For this review, take the finished solid that the model builds, in its own axes (mm). Face numbers are marked on the shaded views. A direction names the side the tool comes from. Give positions to 0.01 mm unless a question says otherwise; leave off trailing zeros. Order: outer loops, then holes, each group sorted by start corner. A loop starts at its lowest first (then second) coordinate and runs counter-clockwise, first axis right, second up.
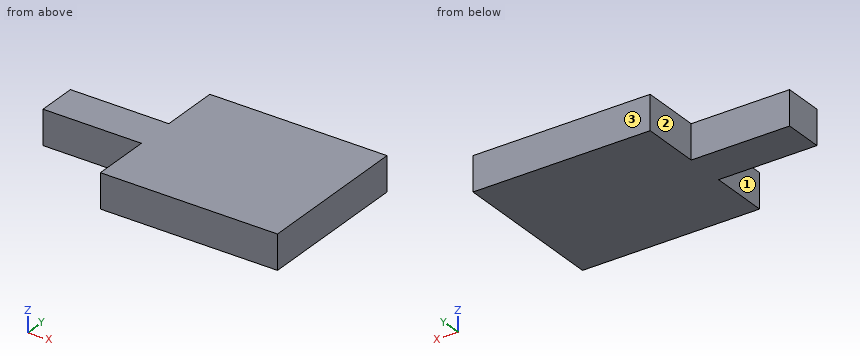
from build123d import *

# Parameters (mm, degrees)
F0_W          = 127
F0_H          = 50.8
F1_DEPTH      = 25.4
F1_DEPTH_BACK = 19.05


with BuildPart() as f1:
    # F0 (on Top) → F1 (new body, two sides)
    with BuildSketch(Plane.XY) as f1_sk:
        Polygon((0, 76.2), (0, 0), (228.6, 0), (228.6, 203.2), (0, 203.2), (0, 127), align=None)
        with Locations((-63.5, 101.6)):
            Rectangle(F0_W, F0_H)
    extrude(amount=F1_DEPTH)
    extrude(f1_sk.sketch, amount=-F1_DEPTH_BACK)


solid = f1.part
1) We need section C-C on y = 65.5. Give the boundary of the cut face in (x, z), then the cut area to 3 significant figures.
Answer sheet:
outline: (0, -19.05) - (228.6, -19.05) - (228.6, 25.4) - (0, 25.4) - close
area: 10,200 mm2
2) To check wall thickness, follow line 1 (X direction, y = 30.5, z = 12); line 2 (Y direction, x = -106.5, z = -5). State the ranges of each line that lie inside material, in increasing order.
Answer sheet:
line 1: x = 0 to 228.6
line 2: y = 76.2 to 127
3) We need section B-B on x = -20.5. Give the boundary of the cut face in (y, z), then the cut area to 3 significant figures.
Answer sheet:
outline: (76.2, -19.05) - (127, -19.05) - (127, 25.4) - (76.2, 25.4) - close
area: 2,260 mm2
4) We need section A-A on z = -3. Give the boundary of the cut face in (x, y).
Answer sheet:
outline: (-127, 76.2) - (0, 76.2) - (0, 0) - (228.6, 0) - (228.6, 203.2) - (0, 203.2) - (0, 127) - (-127, 127) - close
5) Tool access review of the marked faces 1, 2 and 3: name each direction out of +Z, -Z, +X, -X, +Y, -Y from which nothing blocks a thin tool from reaching the whole face with its end or side.
Answer sheet:
face 1: +Z, -Z, -X, -Y
face 2: +Z, -Z, -X, +Y
face 3: +Z, -Z, +X, -X, +Y
6) Clearance check with flat-ended pins moving along their axes: pin 1 (13.5 mm diameter, centred on x = -47, z = -0.5, fed in from -Y); pin 2 (5 mm diameter, centred on x = -51, z = 19, fed in from +Y); pin 3 (22 mm diameter, centred on y = 38, z = 0, fed in from -X). State where each tip first meets the part, or that it passes through.
Answer sheet:
pin 1: stops at y = 76.2
pin 2: stops at y = 127
pin 3: stops at x = 0
